For this review, take the finished solid that the model builds, in its own axes (mm). Face numbers are marked on the shaded views. A direction names the side the tool comes from. Coordinates: 2 decimals unless noted, no trailing zeros. Write each loop counter-clockwise with the first axis right and the second up, starting at its lowest first coordinate (ties: lowest second). Pieces come first, ordered by that corner, then holes.
1) We need section C-C on x = -34. Write out the cut boundary in (y, z).
2) For the marked faces 5, 6 and 7, list the 3-axis set-ups (+Z, -Z, +X, -X, +Y, -Y) from which the entire face can be reached by the end or side of a thin tool; tool diameter is ignored.
3) Insertion check: P1, Ø5, axis at x = -35, z = -1, coming from the +Y side; P2, Ø4, axis at y = -64, z = -2.5, coming from the +X side (3 decimals); P3, Ø1.5, axis at y = -93.5, z = 1.5, coming from the +X side; P4, Ø4, axis at x = -6.56, y = -104.51, coming from the +Z side. Each pin has a flat end and moves straight along its axis. Give the tip position at first contact, or say it passes through.
4) We need section B-B on y = -142.87. Write out the cut boundary in (x, z), then the cut area to 3 significant figures.
5) We need section D-D on y = -81.5. Write out the cut boundary in (x, z), then the cut area to 3 significant figures.
6) Mouldability with a two-part tool opening along Y and no side actions: class the marked faces 1, 2, 3 and 4 as pulls with the +Y half, pulls with the -Y half, needs draft (parallel to the pull), parting line crosses it, or undercut.
7) To check wall thickness, follow line 1 along Y through (x, z) = (4, 1.35); line 2 along Y through (x, z) = (0.02, -2.25); line 3 along Z through (x, y) = (-36, -86). State the ranges of each line that lie inside material, in increasing order.
8) We need section A-A on y = 8.38. Write out the cut boundary in (x, z), then the cut area to 3 significant figures.
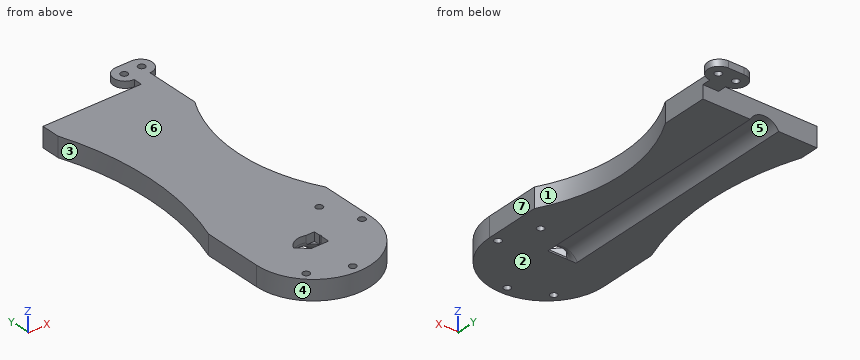
from build123d import *

# Parameters (mm, degrees)
SKETCH_R             = 1.58
PAD_DEPTH            = 3
PAD001_DEPTH         = 6
POCKET_DEPTH         = 4
SKETCH006_R          = 1.58
POCKET001_DEPTH      = 6.001
POCKET001_DEPTH_BACK = -3.001
POCKET002_DEPTH      = 6.001
POCKET002_DEPTH_BACK = -3.001


with BuildPart() as part:
    # Sketch → Pad (new body)
    with BuildSketch(Plane.XY):
        with BuildLine():
            ThreePointArc((-3.6, 13.56), (-8.78, 8.38), (-3.6, 3.2))
            Line((-3.6, 3.2), (-3.6, 0))
            Line((-3.6, 0), (-3.6, -0.8))
            Line((-48.5, -0.8), (-3.6, -0.8))
            Line((-48.5, -0.8), (-48.5, -120.8))
            ThreePointArc((-48.5, -120.8), (-22.45, -146.85), (3.6, -120.8))
            Line((3.6, 0), (3.6, -120.8))
            Line((3.6, 3.2), (3.6, 0))
            ThreePointArc((3.6, 3.2), (8.78, 8.38), (3.6, 13.56))
            Line((3.6, 13.56), (0, 13.56))
            Line((-3.6, 13.56), (0, 13.56))
        make_face()
        with Locations((-4, 8.38)):
            Circle(SKETCH_R, mode=Mode.SUBTRACT)
        with Locations((4, 8.38)):
            Circle(SKETCH_R, mode=Mode.SUBTRACT)
    extrude(amount=PAD_DEPTH)

    # Sketch001 → Pad001 (join)
    with BuildSketch(Plane.XY):
        with BuildLine():
            Line((3.6, -0.8), (-48.5, -0.8))
            Line((-48.5, -0.8), (-48.5, -120.8))
            ThreePointArc((-48.5, -120.8), (-22.45, -146.85), (3.6, -120.8))
            Line((3.6, -0.8), (3.6, -120.8))
        make_face()
    extrude(amount=-PAD001_DEPTH)

    # SubtractivePipe: sweep along a path in Sketch004
    with BuildLine(Plane.YZ) as subtractivepipe_path:
        Line((0, -6), (-114, -6))
        ThreePointArc((-114, -6), (-118.242641, -4.242641), (-120, 0))
        Line((-120, 0), (-120, 3))
    # Sketch002 → SubtractivePipe (sweep, cut)
    with BuildSketch(Plane.XZ):
        with BuildLine():
            Line((-24.5, -6.04), (-31, -6.04))
            ThreePointArc((-18, -6.04), (-24.5, -2.04), (-31, -6.04))
            Line((-24.5, -6.04), (-18, -6.04))
        make_face()
    sweep(path=subtractivepipe_path.line, mode=Mode.SUBTRACT)

    # Sketch005 → Pocket (cut)
    with BuildSketch(Plane.XY.offset(3)):
        Polygon((-26.45, -124.4), (-18.45, -124.4), (-18.45, -116.4), (-26.45, -116.4), (-27.691676, -116.776802), (-31, -120.04), align=None)
    extrude(amount=-POCKET_DEPTH, mode=Mode.SUBTRACT)

    # Sketch006 → Pocket001 (cut, two sides)
    with BuildSketch(Plane.XY) as pocket001_sk:
        with Locations((-22.45, -142.87)):
            Circle(SKETCH006_R)
        with Locations((0.02, -120.4)):
            Circle(SKETCH006_R)
        with Locations((-6.561311, -104.511311)):
            Circle(SKETCH006_R)
        with Locations((-38.338689, -136.288689)):
            Circle(SKETCH006_R)
    extrude(amount=-POCKET001_DEPTH, mode=Mode.SUBTRACT)
    extrude(pocket001_sk.sketch, amount=-POCKET001_DEPTH_BACK, mode=Mode.SUBTRACT)

    # Sketch007 → Pocket002 (cut, two sides)
    with BuildSketch(Plane.XY) as pocket002_sk:
        with BuildLine():
            Line((-58.822819, 0), (-58.822819, -99.491015))
            Line((-58.822819, -99.491015), (-50.649527, -99.491015))
            ThreePointArc((-50.649527, -99.491015), (-41.14496, -49.579042), (-52.256237, 0))
            Line((-52.256237, 0), (-52.256237, 31.290133))
            Line((-52.256237, 31.290133), (11.992633, 31.290133))
            Line((11.992633, -10.093772), (11.992633, 31.290133))
            ThreePointArc((11.992633, -10.093772), (-6.175004, -57.263804), (10.086987, -105.124252))
            Line((35.256332, -105.124252), (10.086987, -105.124252))
            Line((35.256332, 66.325943), (35.256332, -105.124252))
            Line((-58.822819, 66.325943), (35.256332, 66.325943))
            Line((-58.822819, 0), (-58.822819, 66.325943))
        make_face()
    extrude(amount=-POCKET002_DEPTH, mode=Mode.SUBTRACT)
    extrude(pocket002_sk.sketch, amount=-POCKET002_DEPTH_BACK, mode=Mode.SUBTRACT)


solid = part.part
Result:
1. outline: (-144.15, -6) - (-0.8, -6) - (-0.8, 3) - (-144.15, 3) - close
2. face 5: -Z, +Y
2. face 6: +Z, +X, -X, +Y, -Y
2. face 7: +Z, -Z, +X, -Y
3. P1: stops at y = -0.8
3. P2: stops at x = -5.835
3. P3: stops at x = 2.85
3. P4: stops at z = 3
4. outline: (-36.29, -6) - (-24.03, -6) - (-24.03, 3) - (-36.29, 3) - close; (-20.87, -6) - (-8.61, -6) - (-8.61, 3) - (-20.87, 3) - close
4. area: 221 mm2
5. outline: (-44.75, -6) - (-30.98, -6) arc R7.28 cw to (-18.02, -6) - (-2.62, -6) - (-2.62, 3) - (-44.75, 3) - close
5. area: 343 mm2
6. face 1: undercut
6. face 2: needs draft
6. face 3: undercut
6. face 4: pulls with the -Y half
7. line 1: y = 3.22 to 6.8, 9.96 to 13.54
7. line 2: y = -133.98 to -121.98, -118.82 to -88.47, -29.04 to -0.8
7. line 3: z = -6 to 3
8. outline: (-8.78, 0) - (-5.58, 0) - (-5.58, 3) - (-8.78, 3) - close; (-2.42, 0) - (2.42, 0) - (2.42, 3) - (-2.42, 3) - close; (5.58, 0) - (8.78, 0) - (8.78, 3) - (5.58, 3) - close
8. area: 33.7 mm2
